CAD build for the part. Positions are in the model's coordinates, mm. A direction names the side the tool comes from. Coordinates: 2 decimals unless noted, no trailing zeros. Loops run counter-clockwise (first coordinate to the right, second up) from the corner with the lowest first, then second, coordinate; pieces in that order, holes last. Notation, with made-up numbers: (-35.75, 3.5) - (-17.75, 3.5) arc R20 ccw to (-17.75, 41.5) - close; hole circle Ø1 at (9.25, -3). An arc over 180 degrees is marked (long way). Put each result on its own line as item: value.
```python
from build123d import *

# Parameters (mm, degrees)
PAD_DEPTH = 3.3
FILLET_R  = 1


with BuildPart() as part:
    # Sketch002 → Pad (new body)
    with BuildSketch(Plane.XZ):
        with BuildLine():
            Line((16.6, 3.3), (19.9, 3.3))
            Line((19.9, 3.3), (19.9, -24.4))
            ThreePointArc((19.9, -24.4), (25.357643, -30.6783), (32.334399, -26.147541))
            Line((32.334399, -26.147541), (38.398421, -4.999784))
            ThreePointArc((38.398421, -4.999784), (38.488761, 0.175809), (35.979202, 4.703174))
            Line((35.979202, 4.703174), (38.353023, 6.995546))
            ThreePointArc((41.570585, -5.909387), (41.690737, 0.974151), (38.353023, 6.995546))
            Line((35.506563, -27.057144), (41.570585, -5.909387))
            ThreePointArc((16.6, -24.4), (24.898371, -33.946184), (35.506563, -27.057144))
            Line((16.6, 0), (16.6, -24.4))
            Line((3.3, 0), (16.6, 0))
            Line((3.3, -2), (3.3, 0))
            Line((0, -2), (3.3, -2))
            Line((0, 0), (0, -2))
            Line((0, 3.3), (0, 0))
            Line((16.6, 3.3), (0, 3.3))
        make_face()
    extrude(amount=PAD_DEPTH)

    # Fillet
    fillet_edges = [part.edges().sort_by_distance(p)[0] for p in [
        (0, -1.65, 3.3),
        (19.9, -1.65, 3.3),
        (35.979202, -1.65, 4.703174),
        (38.353023, -1.65, 6.995546),
        (37.166113, 0, 5.84936),
        (37.166113, -3.3, 5.84936),
    ]]
    fillet(fillet_edges, radius=FILLET_R)


solid = part.part
```
Q1. Slice it at C-C, the plane x = 11. Give the cut face in (y, z), then the cut area to 3 significant figures.
Determined:
outline: (-3.3, 0) - (0, 0) - (0, 3.3) - (-3.3, 3.3) - close
area: 10.9 mm2
Q2. Wall check: L1, parallel to Z at x = 5, y = -2.7; L2, parallel to X at y = -0.5, z = -27; L3, parallel to X at y = -2.85, z = 1. Give the ranges that are in metal, low to high. Write a range as from..to.
Determined:
L1: 0..3.3
L2: 16.96..20.46, 32.02..35.52
L3: 0..19.9, 38.25..41.68
Q3. Tool access for faces 4 (the flat face through (10, -2, 3.3)), 5 (the cylindrical face through (38.6, -1.63, -0.33)), 6 (the flat face through (10, -2, 0)), 7 (the flat face through (2, -2, -2)), 8 (the flat face through (19.9, -2, -11)): list every direction of +Z, -Z, +X, -X, +Y, -Y with a clear straight run to the whole face (end or side of a thin tool).
Determined:
face 4: +Z, -X, +Y, -Y
face 5: +Y, -Y
face 6: -Z, +Y, -Y
face 7: -Z, -X, +Y, -Y
face 8: +Z, +Y, -Y
Q4. Slice it at A-A, the plane y = -1.75. Give the cut face in (x, z), then the cut area to 3 significant figures.
Determined:
outline: (0, -2) - (3.3, -2) - (3.3, 0) - (16.6, 0) - (16.6, -24.4) arc R9.64 ccw to (35.51, -27.06) - (41.57, -5.91) arc R13.3 ccw to (39.07, 6.19) arc R1 ccw to (37.6, 6.27) - (36.67, 5.37) arc R1 ccw to (36.58, 4.02) arc R10 cw to (38.4, -5) - (32.33, -26.15) arc R6.34 cw to (19.9, -24.4) - (19.9, 2.3) arc R1 ccw to (18.9, 3.3) - (1, 3.3) arc R1 ccw to (0, 2.3) - close
area: 340 mm2
Q5. Mould opens along X. For faces 1 (the flat face through (19.6, -3.3, -12.3)), 2 (the cylindrical face through (37.44, -0.187, 5.534)), 3 (the flat face through (35.324, -1.627, -15.722)) say: +X half, -X half, draft (parallel to the pull), parting line (faces both ways), or undercut.
Determined:
face 1: draft
face 2: -X half
face 3: undercut
Q6. Slice it at D-D, the plane x = 24.5. Give the cut face in (y, z), then the cut area to 3 significant figures.
Determined:
outline: (-3.3, -33.88) - (0, -33.88) - (0, -30.5) - (-3.3, -30.5) - close
area: 11.2 mm2
Q7. Slice it at B-B, the plane z = -13.5. Give the cut face in (x, y), then the cut area to 3 significant figures.
Determined:
outline: (16.6, -3.3) - (19.9, -3.3) - (19.9, 0) - (16.6, 0) - close; (35.96, -3.3) - (39.39, -3.3) - (39.39, 0) - (35.96, 0) - close
area: 22.2 mm2
Q8. Pin check, flat tips, straight feed: pin 1 Ø0.6 at (y, z) = (-1.5, -0.5) entering from +X; pin 2 Ø1 at (y, z) = (-2.5, -15) entering from +X; pin 3 Ø1.6 at (x, y) = (11, -1.5) entering from -Z. Stop position of each tip, or through.
Determined:
pin 1: x = 42.01
pin 2: x = 39.11
pin 3: z = 0
